```python
from build123d import *

# Parameters (mm, degrees)
SKETCH1_R               = 2
BOSS_EXTRUDE1_DEPTH     = 10
SKETCH2_R               = 5
CUT_EXTRUDE1_DEPTH      = 33
CUT_EXTRUDE1_DEPTH_BACK = 33
SKETCH3_R               = 7.5
CUT_EXTRUDE2_DEPTH      = 16
SKETCH4_R               = 3.5
CUT_EXTRUDE3_DEPTH      = 8
CUT_EXTRUDE4_DEPTH      = 7
BOSS_EXTRUDE2_START     = -10
BOSS_EXTRUDE2_DEPTH     = 7
LPATTERN1_COUNT         = 6
LPATTERN1_PITCH         = 2
LPATTERN2_COUNT         = 2
LPATTERN2_PITCH         = 52.6
LPATTERN2_START         = -10
LPATTERN2_COPY_1_DEPTH  = 7
LPATTERN2_COPY_2_DEPTH  = 7
LPATTERN2_COPY_3_DEPTH  = 7
LPATTERN2_COPY_4_DEPTH  = 7
LPATTERN2_COPY_5_DEPTH  = 7
FILLET1_R               = 5
FILLET2_R               = 1
SKETCH8_R               = 2
BOSS_EXTRUDE3_DEPTH     = 3


with BuildPart() as part:
    # Sketch1 → Boss-Extrude1 (new body)
    with BuildSketch(Plane.XY):
        with BuildLine():
            Line((-27, -21.25), (27, -21.25))
            ThreePointArc((27, -21.25), (30.771278101, -19.532904428), (31.952298231, -15.560984594))
            Line((31.952298231, -15.560984594), (27.952298231, 13.189015406))
            ThreePointArc((27.952298231, 13.189015406), (26.282904428, 16.271278101), (23, 17.5))
            Line((23, 17.5), (-23, 17.5))
            ThreePointArc((-23, 17.5), (-26.282904428, 16.271278101), (-27.952298231, 13.189015406))
            Line((-27.952298231, 13.189015406), (-31.952298231, -15.560984594))
            ThreePointArc((-31.952298231, -15.560984594), (-30.771278101, -19.532904428), (-27, -21.25))
        make_face()
        with Locations((-10, -16.25)):
            Circle(SKETCH1_R, mode=Mode.SUBTRACT)
        with Locations((10, -16.25)):
            Circle(SKETCH1_R, mode=Mode.SUBTRACT)
        with Locations((23, 12.5)):
            Circle(SKETCH1_R, mode=Mode.SUBTRACT)
        with Locations((-23, 12.5)):
            Circle(SKETCH1_R, mode=Mode.SUBTRACT)
    extrude(amount=BOSS_EXTRUDE1_DEPTH)

    # Sketch2 → Cut-Extrude1 (cut, two sides)
    with BuildSketch(Plane(origin=(0, 0, 0), x_dir=(0, 0, -1), z_dir=(1, 0, 0))) as cut_extrude1_sk:
        with Locations((1.5, 0)):
            Circle(SKETCH2_R)
    extrude(amount=CUT_EXTRUDE1_DEPTH, mode=Mode.SUBTRACT)
    extrude(cut_extrude1_sk.sketch, amount=-CUT_EXTRUDE1_DEPTH_BACK, mode=Mode.SUBTRACT)

    # Sketch3 → Cut-Extrude2 (cut)
    with BuildSketch(Plane(origin=(15, 0, 0), x_dir=(0, 0, -1), z_dir=(1, 0, 0))):
        with Locations((1.5, 0)):
            Circle(SKETCH3_R)
    cut_extrude2 = extrude(amount=CUT_EXTRUDE2_DEPTH, mode=Mode.SUBTRACT)

    # Mirror1: Cut-Extrude2 across plane
    add(cut_extrude2.mirror(Plane(origin=(0, 0, 0), x_dir=(0, 0, 1), z_dir=(1, 0, 0))), mode=Mode.SUBTRACT)

    # Sketch4 → Cut-Extrude3 (cut)
    with BuildSketch(Plane.XY.offset(10)):
        with Locations((10, -16.25)):
            Circle(SKETCH4_R)
        with Locations((-10, -16.25)):
            Circle(SKETCH4_R)
        with Locations((23, 12.5)):
            Circle(SKETCH4_R)
        with Locations((-23, 12.5)):
            Circle(SKETCH4_R)
    extrude(amount=-CUT_EXTRUDE3_DEPTH, mode=Mode.SUBTRACT)

    # Sketch6 → Cut-Extrude4 (cut)
    with BuildSketch(Plane(origin=(0, 0, 0), x_dir=(-1, 0, 0), z_dir=(0, 0, -1))):
        Polygon((-31.974937186, -15.75), (-20.589119642, -15.75), (-14.48075081, -21.25), (-12.08958833, -21.25), (-19.974937186, -14.15), (-31.974937186, -14.15), align=None)
        Polygon((20.589119642, -15.75), (14.48075081, -21.25), (12.08958833, -21.25), (19.974937186, -14.15), (31.974937186, -14.15), (31.974937186, -15.75), align=None)
    extrude(amount=-CUT_EXTRUDE4_DEPTH, mode=Mode.SUBTRACT)

    # Sketch7 → Boss-Extrude2 (add)
    with BuildSketch(Plane.XY.offset(10).offset(BOSS_EXTRUDE2_START)):
        with BuildLine():
            Line((30.724937186, -15.75), (31.924937186, -15.75))
            Line((31.924937186, -15.75), (31.924937186, -15.55))
            ThreePointArc((31.924937186, -15.55), (31.324937186, -14.95), (30.724937186, -15.55))
            Line((30.724937186, -15.55), (30.724937186, -15.75))
        make_face()
    boss_extrude2 = extrude(amount=BOSS_EXTRUDE2_DEPTH)

    # LPattern1: Boss-Extrude2 ×6
    with Locations(*[(-i * LPATTERN1_PITCH, 0, 0) for i in range(1, LPATTERN1_COUNT)]):
        add(boss_extrude2)

    # LPattern2: Boss-Extrude2 ×2
    with Locations(*[(-i * LPATTERN2_PITCH, 0, 0) for i in range(1, LPATTERN2_COUNT)]):
        add(boss_extrude2)

    # LPattern2 copy 1 sketch → LPattern2 copy 1 (add)
    with BuildSketch(Plane(origin=(-54.6, 0, 10), x_dir=(1, 0, 0), z_dir=(0, 0, 1)).offset(LPATTERN2_START)):
        with BuildLine():
            Line((30.724937186, -15.75), (31.924937186, -15.75))
            Line((31.924937186, -15.75), (31.924937186, -15.55))
            ThreePointArc((31.924937186, -15.55), (31.324937186, -14.95), (30.724937186, -15.55))
            Line((30.724937186, -15.55), (30.724937186, -15.75))
        make_face()
    extrude(amount=LPATTERN2_COPY_1_DEPTH)

    # LPattern2 copy 2 sketch → LPattern2 copy 2 (add)
    with BuildSketch(Plane(origin=(-56.6, 0, 10), x_dir=(1, 0, 0), z_dir=(0, 0, 1)).offset(LPATTERN2_START)):
        with BuildLine():
            Line((30.724937186, -15.75), (31.924937186, -15.75))
            Line((31.924937186, -15.75), (31.924937186, -15.55))
            ThreePointArc((31.924937186, -15.55), (31.324937186, -14.95), (30.724937186, -15.55))
            Line((30.724937186, -15.55), (30.724937186, -15.75))
        make_face()
    extrude(amount=LPATTERN2_COPY_2_DEPTH)

    # LPattern2 copy 3 sketch → LPattern2 copy 3 (add)
    with BuildSketch(Plane(origin=(-58.6, 0, 10), x_dir=(1, 0, 0), z_dir=(0, 0, 1)).offset(LPATTERN2_START)):
        with BuildLine():
            Line((30.724937186, -15.75), (31.924937186, -15.75))
            Line((31.924937186, -15.75), (31.924937186, -15.55))
            ThreePointArc((31.924937186, -15.55), (31.324937186, -14.95), (30.724937186, -15.55))
            Line((30.724937186, -15.55), (30.724937186, -15.75))
        make_face()
    extrude(amount=LPATTERN2_COPY_3_DEPTH)

    # LPattern2 copy 4 sketch → LPattern2 copy 4 (add)
    with BuildSketch(Plane(origin=(-60.6, 0, 10), x_dir=(1, 0, 0), z_dir=(0, 0, 1)).offset(LPATTERN2_START)):
        with BuildLine():
            Line((30.724937186, -15.75), (31.924937186, -15.75))
            Line((31.924937186, -15.75), (31.924937186, -15.55))
            ThreePointArc((31.924937186, -15.55), (31.324937186, -14.95), (30.724937186, -15.55))
            Line((30.724937186, -15.55), (30.724937186, -15.75))
        make_face()
    extrude(amount=LPATTERN2_COPY_4_DEPTH)

    # LPattern2 copy 5 sketch → LPattern2 copy 5 (add)
    with BuildSketch(Plane(origin=(-62.6, 0, 10), x_dir=(1, 0, 0), z_dir=(0, 0, 1)).offset(LPATTERN2_START)):
        with BuildLine():
            Line((30.724937186, -15.75), (31.924937186, -15.75))
            Line((31.924937186, -15.75), (31.924937186, -15.55))
            ThreePointArc((31.924937186, -15.55), (31.324937186, -14.95), (30.724937186, -15.55))
            Line((30.724937186, -15.55), (30.724937186, -15.75))
        make_face()
    extrude(amount=LPATTERN2_COPY_5_DEPTH)

    # Fillet1
    fillet1_edges = [part.edges().sort_by_distance(p)[0] for p in [
        (12.08958833, -21.25, 3.5),
        (-12.08958833, -21.25, 3.5),
    ]]
    fillet(fillet1_edges, radius=FILLET1_R)

    # Fillet2
    fillet2_edges = [part.edges().sort_by_distance(p)[0] for p in [
        (14.48075081, -21.25, 3.5),
        (-14.48075081, -21.25, 3.5),
    ]]
    fillet(fillet2_edges, radius=FILLET2_R)

    # Sketch8 → Boss-Extrude3 (add)
    with BuildSketch(Plane(origin=(0, 0, 0), x_dir=(-1, 0, 0), z_dir=(0, 0, -1))):
        with BuildLine():
            Line((-31.924937186, -15.75), (-31.974937186, -15.75))
            ThreePointArc((-31.974937186, -15.75), (-30.708099244, -19.604101966), (-27, -21.25))
            Line((-27, -21.25), (-17.085839875, -21.25))
            ThreePointArc((-17.085839875, -21.25), (-16.152259448, -20.60836795), (-16.416709268, -19.506855175))
            Line((-16.416709268, -19.506855175), (-20.589119642, -15.75))
            Line((-20.589119642, -15.75), (-20.724937186, -15.75))
            Line((-20.724937186, -15.75), (-20.724937186, -15.55))
            ThreePointArc((-20.724937186, -15.55), (-21.324937186, -14.95), (-21.924937186, -15.55))
            Line((-21.924937186, -15.55), (-21.924937186, -15.75))
            Line((-21.924937186, -15.75), (-22.724937186, -15.75))
            Line((-22.724937186, -15.75), (-22.724937186, -15.55))
            ThreePointArc((-22.724937186, -15.55), (-23.324937186, -14.95), (-23.924937186, -15.55))
            Line((-23.924937186, -15.55), (-23.924937186, -15.75))
            Line((-23.924937186, -15.75), (-24.724937186, -15.75))
            Line((-24.724937186, -15.75), (-24.724937186, -15.55))
            ThreePointArc((-24.724937186, -15.55), (-25.324937186, -14.95), (-25.924937186, -15.55))
            Line((-25.924937186, -15.55), (-25.924937186, -15.75))
            Line((-25.924937186, -15.75), (-26.724937186, -15.75))
            Line((-26.724937186, -15.75), (-26.724937186, -15.55))
            ThreePointArc((-26.724937186, -15.55), (-27.324937186, -14.95), (-27.924937186, -15.55))
            Line((-27.924937186, -15.55), (-27.924937186, -15.75))
            Line((-27.924937186, -15.75), (-28.724937186, -15.75))
            Line((-28.724937186, -15.75), (-28.724937186, -15.55))
            ThreePointArc((-28.724937186, -15.55), (-29.324937186, -14.95), (-29.924937186, -15.55))
            Line((-29.924937186, -15.55), (-29.924937186, -15.75))
            Line((-29.924937186, -15.75), (-30.724937186, -15.75))
            Line((-30.724937186, -15.75), (-30.724937186, -15.55))
            ThreePointArc((-30.724937186, -15.55), (-31.324937186, -14.95), (-31.924937186, -15.55))
            Line((-31.924937186, -15.55), (-31.924937186, -15.75))
        make_face()
        with BuildLine():
            Line((-31.755987331, -14.15), (-19.974937186, -14.15))
            Line((-19.974937186, -14.15), (-13.515921187, -19.965724127))
            ThreePointArc((-13.515921187, -19.965724127), (-11.962107903, -20.917902132), (-10.170268155, -21.25))
            Line((-10.170268155, -21.25), (10.170268155, -21.25))
            ThreePointArc((10.170268155, -21.25), (11.962107903, -20.917902132), (13.515921187, -19.965724127))
            Line((13.515921187, -19.965724127), (19.974937186, -14.15))
            Line((19.974937186, -14.15), (31.755987331, -14.15))
            Line((31.755987331, -14.15), (31.35250907, -11.25))
            Line((31.35250907, -11.25), (-31.35250907, -11.25))
            Line((-31.35250907, -11.25), (-31.755987331, -14.15))
        make_face()
        with Locations((-10, -16.25)):
            Circle(SKETCH8_R, mode=Mode.SUBTRACT)
        with Locations((10, -16.25)):
            Circle(SKETCH8_R, mode=Mode.SUBTRACT)
        with BuildLine():
            Line((21.875062814, -15.75), (21.875062814, -15.55))
            ThreePointArc((21.875062814, -15.55), (21.275062814, -14.95), (20.675062814, -15.55))
            Line((20.675062814, -15.55), (20.675062814, -15.75))
            Line((20.675062814, -15.75), (20.589119642, -15.75))
            Line((20.589119642, -15.75), (16.416709268, -19.506855175))
            ThreePointArc((16.416709268, -19.506855175), (16.152259448, -20.60836795), (17.085839875, -21.25))
            Line((17.085839875, -21.25), (27, -21.25))
            ThreePointArc((27, -21.25), (30.708099244, -19.604101966), (31.974937186, -15.75))
            Line((31.974937186, -15.75), (31.875062814, -15.75))
            Line((31.875062814, -15.75), (31.875062814, -15.55))
            ThreePointArc((31.875062814, -15.55), (31.275062814, -14.95), (30.675062814, -15.55))
            Line((30.675062814, -15.55), (30.675062814, -15.75))
            Line((30.675062814, -15.75), (29.875062814, -15.75))
            Line((29.875062814, -15.75), (29.875062814, -15.55))
            ThreePointArc((29.875062814, -15.55), (29.275062814, -14.95), (28.675062814, -15.55))
            Line((28.675062814, -15.55), (28.675062814, -15.75))
            Line((28.675062814, -15.75), (27.875062814, -15.75))
            Line((27.875062814, -15.75), (27.875062814, -15.55))
            ThreePointArc((27.875062814, -15.55), (27.275062814, -14.95), (26.675062814, -15.55))
            Line((26.675062814, -15.55), (26.675062814, -15.75))
            Line((26.675062814, -15.75), (25.875062814, -15.75))
            Line((25.875062814, -15.75), (25.875062814, -15.55))
            ThreePointArc((25.875062814, -15.55), (25.275062814, -14.95), (24.675062814, -15.55))
            Line((24.675062814, -15.55), (24.675062814, -15.75))
            Line((24.675062814, -15.75), (23.875062814, -15.75))
            Line((23.875062814, -15.75), (23.875062814, -15.55))
            ThreePointArc((23.875062814, -15.55), (23.275062814, -14.95), (22.675062814, -15.55))
            Line((22.675062814, -15.55), (22.675062814, -15.75))
            Line((22.675062814, -15.75), (21.875062814, -15.75))
        make_face()
    extrude(amount=BOSS_EXTRUDE3_DEPTH)


solid = part.part
```
The model under review builds one solid part; all positions refer to its coordinate system, in mm. A direction names the side the tool comes from. Give positions to 0.01 mm unless a question says otherwise; leave off trailing zeros. Write each loop counter-clockwise with the first axis right and the second up, starting at its lowest first coordinate (ties: lowest second). Pieces come first, ordered by that corner, then holes. Notation, with made-up numbers: (53.5, 33.25) -> (74.5, 33.25) arc R30 ccw to (74.5, 62.25) -> close; hole circle Ø7 at (8, -7). An arc over 180 degrees is marked (long way). Answer in a Markdown table with one row per item.
1) Add section C-C on y = 2. State the section outline as (x, z) points.
Worked answers:
| item | result |
|---|---|
| outline | (-29.51, 5.73) -> (-15, 5.73) -> (-15, 3.08) -> (15, 3.08) -> (15, 5.73) -> (29.51, 5.73) -> (29.51, 10) -> (-29.51, 10) -> close |
2) Tool access review of faces 4 (the cylindrical face through (-29.26, -14.95, 1.93)), 5 (the flat face through (15, 0, 4)), 6 (the cylindrical face through (21.526, 13.852, 0.986)), 7 (the flat face through (24, -18, -3)), 8 (the flat face through (12, -18, 2)): name each direction out of +Z, -Z, +X, -X, +Y, -Y from which nothing blocks a thin tool from reaching the whole face with its end or side.
Worked answers:
| item | result |
|---|---|
| face 4 | -Z |
| face 5 | -Z, +X |
| face 6 | +Z, -Z |
| face 7 | -Z, +X, -X, +Y, -Y |
| face 8 | +Z |
3) Add section B-B on z = 9.25. State the section outline as (x, y) points.
Worked answers:
| item | result |
|---|---|
| outline | (-31.95, -15.56) arc R5 ccw to (-27, -21.25) -> (27, -21.25) arc R5 ccw to (31.95, -15.56) -> (27.95, 13.19) arc R5 ccw to (23, 17.5) -> (-23, 17.5) arc R5 ccw to (-27.95, 13.19) -> close; hole circle Ø7 at (-23, 12.5); hole circle Ø7 at (-10, -16.25); hole circle Ø7 at (10, -16.25); hole circle Ø7 at (23, 12.5) |
4) Mouldability with a two-part tool opening along X and no side actions: class faces 1 (the cylindrical face through (-26.245, 16.304, 4.93)), 2 (the cylindrical face through (0.2, 0.1, 3.5)), 3 (the cylindrical face through (-25.26, -14.95, 1.93)) as +X half, -X half, draft (parallel to the pull), parting line (faces both ways), or undercut.
Worked answers:
| item | result |
|---|---|
| face 1 | -X half |
| face 2 | draft |
| face 3 | undercut |
5) Clearance check with flat-ended pins moving along their axes: P1, Ø2, axis at x = 14.5, z = 2, coming from the -Y side; P2, Ø2.5, axis at x = 10, y = -16.25, coming from the -Z side; P3, Ø3.5, axis at x = -18, y = -16.5, coming from the -Z side; P4, Ø6, axis at y = 9, z = 8, coming from the +X side. State where each tip first meets the part, or that it passes through.
Worked answers:
| item | result |
|---|---|
| P1 | y = -19.98 |
| P2 | through |
| P3 | z = -3 |
| P4 | x = 28.95 |
6) For L1, parallel to Y at x = -23, z = 7.25; L2, parallel to X at y = -16.25, z = -1.8; L3, parallel to Y at x = -10, z = 6.5, list the stretches that pass through material, from the lowest coordinate up. Write a range as [from, to].
Worked answers:
| item | result |
|---|---|
| L1 | [-21.25, 9], [16, 17.5] |
| L2 | [-32, -20.03], [-17.64, -12], [-8, 8], [12, 17.64], [20.03, 32] |
| L3 | [-21.25, -19.75], [-12.75, 17.5] |
7) Add section A-A on y = 11.5. State the section outline as (x, z) points, plus the area to 3 significant figures.
Worked answers:
| item | result |
|---|---|
| outline | (-28.19, 0) -> (-24.73, 0) -> (-24.73, 2) -> (-26.35, 2) -> (-26.35, 10) -> (-28.19, 10) -> close; (-21.27, 0) -> (21.27, 0) -> (21.27, 2) -> (19.65, 2) -> (19.65, 10) -> (-19.65, 10) -> (-19.65, 2) -> (-21.27, 2) -> close; (24.73, 0) -> (28.19, 0) -> (28.19, 10) -> (26.35, 10) -> (26.35, 2) -> (24.73, 2) -> close |
| area | 443 mm² |
